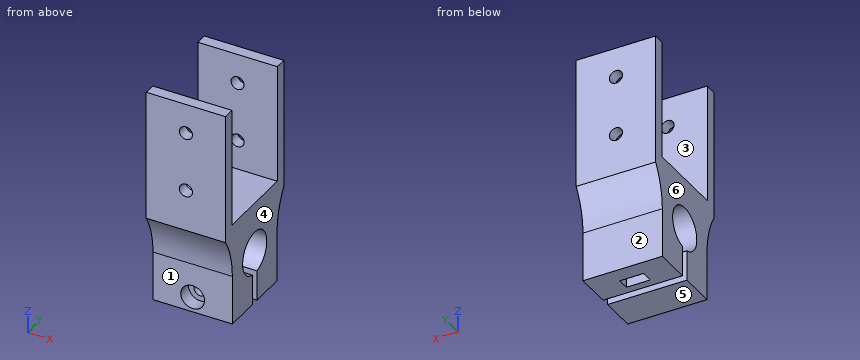
```python
from build123d import *

# Parameters (mm, degrees)
SKETCH_2_W          = 20
SKETCH_2_H          = 26
EXTRUDE_1_DEPTH     = 3
SKETCH_3_W          = 20
SKETCH_3_H          = 2.9
EXTRUDE_2_DEPTH     = 30
SKETCH_4_R          = 1.65
CUT_EXTRUDE_1_DEPTH = 23.1
SKETCH_5_W          = 20
SKETCH_5_H          = 20
EXTRUDE_3_DEPTH     = 20
SKETCH_6_R          = 5.4
CUT_EXTRUDE_2_DEPTH = 20
CUT_EXTRUDE_3_DEPTH = 20
SKETCH_8_W          = 20
SKETCH_8_H          = 9
EXTRUDE_4_DEPTH     = 3
SKETCH_9_R          = 1.65
CUT_EXTRUDE_4_DEPTH = 16
SKETCH_10_R         = 3
CUT_EXTRUDE_5_DEPTH = 3.5
CUT_EXTRUDE_START   = -2
CUT_EXTRUDE_6_DEPTH = 3
SKETCH_12_R         = 1.65
CUT_EXTRUDE_7_DEPTH = 2
FILLET_1_R          = 20


with BuildPart() as part:
    # Эскиз2 → Бобышка-Вытянуть1 (new body)
    with BuildSketch(Plane.XY):
        Rectangle(SKETCH_2_W, SKETCH_2_H)
    extrude(amount=EXTRUDE_1_DEPTH)

    # Эскиз3 → Бобышка-Вытянуть2 (add)
    with BuildSketch(Plane.XY.offset(3)):
        with Locations((0, 11.55)):
            Rectangle(SKETCH_3_W, SKETCH_3_H)
        with Locations((0, -11.55)):
            Rectangle(SKETCH_3_W, SKETCH_3_H)
    extrude(amount=EXTRUDE_2_DEPTH)

    # Эскиз4 → Вырез-Вытянуть1 (cut)
    with BuildSketch(Plane(origin=(0, 13, 0), x_dir=(1, 0, 0), z_dir=(0, 1, 0))):
        with Locations(Location((0, -10.5, 0), (0, 0, 180))):
            Circle(SKETCH_4_R)
        with Locations(Location((0, -25.5, 0), (0, 0, 180))):
            Circle(SKETCH_4_R)
    cut_extrude_1 = extrude(amount=-CUT_EXTRUDE_1_DEPTH, mode=Mode.SUBTRACT)

    # Зеркальное отражение1: Вырез-Вытянуть1 across plane
    add(cut_extrude_1.mirror(Plane.ZX), mode=Mode.SUBTRACT)

    # Эскиз5 → Бобышка-Вытянуть3 (add)
    with BuildSketch(Plane(origin=(0, 0, 0), x_dir=(-1, 0, 0), z_dir=(0, 0, -1))):
        Rectangle(SKETCH_5_W, SKETCH_5_H)
    extrude(amount=EXTRUDE_3_DEPTH)

    # Эскиз6 → Вырез-Вытянуть2 (cut)
    with BuildSketch(Plane(origin=(10, 0, 0), x_dir=(0, 0, -1), z_dir=(1, 0, 0))):
        with Locations(Location((10, 0, 0), (0, 0, 90))):
            Circle(SKETCH_6_R)
    extrude(amount=-CUT_EXTRUDE_2_DEPTH, mode=Mode.SUBTRACT)

    # Эскиз7 → Вырез-Вытянуть3 (cut)
    with BuildSketch(Plane(origin=(10, 0, 0), x_dir=(0, 0, -1), z_dir=(1, 0, 0))):
        with BuildLine():
            Line((15.306599665, 1), (20, 1))
            Line((20, 1), (20, -1))
            Line((20, -1), (15.306599665, -1))
            ThreePointArc((15.306599665, -1), (15.4, 0), (15.306599665, 1))
        make_face()
    extrude(amount=-CUT_EXTRUDE_3_DEPTH, mode=Mode.SUBTRACT)

    # Эскиз8 → Бобышка-Вытянуть4 (add)
    with BuildSketch(Plane(origin=(0, 0, -20), x_dir=(-1, 0, 0), z_dir=(0, 0, -1))):
        with Locations((0, 5.5)):
            Rectangle(SKETCH_8_W, SKETCH_8_H)
        with Locations((0, -5.5)):
            Rectangle(SKETCH_8_W, SKETCH_8_H)
    extrude(amount=EXTRUDE_4_DEPTH)

    # Эскиз9 → Вырез-Вытянуть4 (cut)
    with BuildSketch(Plane.XZ.offset(10)):
        with Locations(Location((0, -19.153299832, 0), (0, 0, 270))):
            Circle(SKETCH_9_R)
    extrude(amount=-CUT_EXTRUDE_4_DEPTH, mode=Mode.SUBTRACT)

    # Эскиз10 → Вырез-Вытянуть5 (cut)
    with BuildSketch(Plane.XZ.offset(10)):
        with Locations(Location((0, -19.153299832, 0), (0, 0, 270))):
            Circle(SKETCH_10_R)
    extrude(amount=-CUT_EXTRUDE_5_DEPTH, mode=Mode.SUBTRACT)

    # Эскиз11 → Вырез-Вытянуть6 (cut)
    with BuildSketch(Plane.XZ.offset(-1).offset(CUT_EXTRUDE_START)):
        Polygon((3, -23), (3, -17.421249025), (0, -15.689198217), (-3, -17.421249025), (-3, -23), align=None)
    extrude(amount=-CUT_EXTRUDE_6_DEPTH, mode=Mode.SUBTRACT)

    # Эскиз12 → Вырез-Вытянуть7 (cut)
    with BuildSketch(Plane.XZ.offset(-6)):
        with Locations(Location((0, -19.153299832, 0), (0, 0, 270))):
            Circle(SKETCH_12_R)
    extrude(amount=-CUT_EXTRUDE_7_DEPTH, mode=Mode.SUBTRACT)

    # Скругление1
    # the kernel refuses this fillet: 20 mm, written as the material it adds along each edge
    with BuildSketch(Plane(origin=(10, -10, 0), x_dir=(0, 0, -1), z_dir=(-1, 0, 0))) as fillet_1_piece_1:
        with BuildLine():
            CenterArc((10.535653753, 20), FILLET_1_R, 238.211669383, 31.788330617)
            Line((0, 3), (0, 0))
            Line((0, 0), (10.535653753, 0))
        make_face()
    extrude(amount=20)
    with BuildSketch(Plane(origin=(-10, 10, 0), x_dir=(0, 1, 0), z_dir=(1, 0, 0))) as fillet_1_piece_2:
        with BuildLine():
            CenterArc((20, -10.535653753), FILLET_1_R, 148.211669383, 31.788330617)
            Line((0, -10.535653753), (0, 0))
            Line((0, 0), (3, 0))
        make_face()
    extrude(amount=20)


solid = part.part
```
Geometry: final body of the model. Coordinates: model frame, mm. Face numbers are marked on the shaded views. A direction names the side the tool comes from. Give positions to 0.01 mm unless a question says otherwise; leave off trailing zeros. Loops run counter-clockwise (first coordinate to the right, second up) from the corner with the lowest first, then second, coordinate; pieces in that order, holes last. Notation, with made-up numbers: (46, -39.75) - (54, -39.75) arc R17 cw to (54, -24.75) - close; hole circle Ø11 at (-29.5, -7.75). An arc over 180 degrees is marked (long way). Answer as CSV lines item,"result". Start each with the question number.
(1) Section query D-D (y = 2). Output: boundary loops of the cut face in (x, z).
(2) Pin query (flat end, axial travel): P1, Ø6.5, axis at x = -0.5, z = -20, coming from the +Y side; P2, Ø1.8, axis at x = -0.5, z = -17.5, coming from the -Y side; P3, Ø2, axis at x = 2, y = -7, coming from the +Z side. Return the tip coordinate at first contact, or that it passes through.
(3) Section query C-C (z = -13). Output: boundary loops of the cut face in (x, y), and give its area (3 significant figures).
(4) Section query B-B (y = -9). Output: boundary loops of the cut face in (x, z), and give its area (3 significant figures).
(5) Reachability of the marked faces 1, 2 and 3 from +Z, -Z, +X, -X, +Y, -Y: full face, straight path, thin tool, end or side. Return the list, or none.
(6) Mould query, pull axis X, two halves, no side actions, for the marked faces 4, 5 and 6. Classes: +X half, -X half, draft (parallel to the pull), parting line (faces both ways), or undercut.
(7) Ray query, line 1 along Y through (x, z) = (-5.75, -18); line 2 along Z through (x, y) = (0.25, -7.75); line 3 along Y through (x, z) = (8, 5.5). Return the intervals inside material, ascending. Write a range as [from, to].
(8) Section query A-A (z = 10.5). Output: boundary loops of the cut face in (x, y).
Worked answers:
1,outline,"(-10, -23) - (10, -23) - (10, -15.02) - (-10, -15.02) - close; (-10, -4.98) - (10, -4.98) - (10, 3) - (-10, 3) - close; hole circle Ø3.3 at (0, -19.15)"
2,P1,"stops at y = 10"
2,P2,"stops at y = -6.5"
2,P3,"stops at z = 3"
3,outline,"(-10, -10) - (10, -10) - (10, -4.49) - (-10, -4.49) - close; (-10, 4.49) - (10, 4.49) - (10, 10) - (-10, 10) - close"
3,area,"220 mm^2"
4,outline,"(-10, -23) - (10, -23) - (10, 3) - (-10, 3) - close; hole circle Ø6 at (0, -19.15)"
4,area,"492 mm^2"
5,face 1,"-Z, +X, -X, -Y"
5,face 2,"-Z, +X, -X, +Y"
5,face 3,"+Z, +X, -X"
6,face 4,"+X half"
6,face 5,"draft"
6,face 6,"-X half"
7,line 1,"y = [-10, -1], [1, 10]"
7,line 2,"z = [-23, -22.14], [-16.16, 3]"
7,line 3,"y = [-13, -10.1], [10.1, 13]"
8,outline,"(-10, -13) - (-1.65, -13) - (-1.65, -10.1) - (-10, -10.1) - close; (-10, 10.1) - (-1.65, 10.1) - (-1.65, 13) - (-10, 13) - close; (1.65, -13) - (10, -13) - (10, -10.1) - (1.65, -10.1) - close; (1.65, 10.1) - (10, 10.1) - (10, 13) - (1.65, 13) - close"
